CAD build for the part. Positions are in the model's coordinates, mm. A direction names the side the tool comes from. Round coordinates to 2 decimals unless told otherwise and drop trailing zeros. Write each loop counter-clockwise with the first axis right and the second up, starting at its lowest first coordinate (ties: lowest second). Pieces come first, ordered by that corner, then holes. Notation, with made-up numbers: (40, -21.5) - (54, -21.5) arc R31 ccw to (54, 9.5) - close; hole circle Ø8 at (-35.5, -36.75). An arc over 180 degrees is marked (long way). Answer in a Markdown table with one row per item.
```python
from build123d import *

# Parameters (mm, degrees)
PAD_DEPTH         = 20
POCKET_DEPTH      = 6.001
POCKET_DEPTH_BACK = -28.001


with BuildPart() as part:
    # AdditivePipe: sweep along a path in Sketch
    with BuildLine(Plane.XY) as additivepipe_path:
        Line((0, 0), (0, 47))
    # Sketch001 → AdditivePipe (sweep)
    with BuildSketch(Plane.XZ):
        Polygon((-20, 6), (-20, -6), (-16, -6), (-9, -6), (9, -6), (16, -6), (20, -6), (20, 6), (16, 6), (16, 3), (9, 3), (9, 6), (-9, 6), (-9, 3), (-16, 3), (-16, 6), align=None)
    sweep(path=additivepipe_path.line)

    # Sketch002 → Pad (new body, symmetric)
    with BuildSketch(Plane.YZ):
        Polygon((47, 3), (47, 14), (34, 28), (22, 28), (22, 14), (29, 14), (29, 3), align=None)
    extrude(amount=PAD_DEPTH, both=True)

    # Sketch003 → Pocket (cut, two sides)
    with BuildSketch(Plane.XY) as pocket_sk:
        with BuildLine():
            Line((-4.5, 0), (4.5, 0))
            Line((4.5, 0), (4.5, 7))
            ThreePointArc((4.5, 7), (0, 19.361903), (-4.5, 7))
            Line((-4.5, 0), (-4.5, 7))
        make_face()
    extrude(amount=-POCKET_DEPTH, mode=Mode.SUBTRACT)
    extrude(pocket_sk.sketch, amount=-POCKET_DEPTH_BACK, mode=Mode.SUBTRACT)


solid = part.part
```
Q1. Pull direction Z, two halves, no side cores. Call faces 5 (the flat face through (0, 24, -6)), 6 (the flat face through (0, 47, 4)), 7 (the flat face through (13, 15, 3)), 8 (the flat face through (0, 28, 28)): released by +Z, released by -Z, zero draft, split by the parting line, or undercut.
Computed:
| item | result |
|---|---|
| face 5 | released by -Z |
| face 6 | zero draft |
| face 7 | undercut |
| face 8 | released by +Z |
Q2. Saw through at B-B on x = 0. List the corners of the cut face in (y, z).
Computed:
| item | result |
|---|---|
| outline | (19.36, -6) - (47, -6) - (47, 14) - (34, 28) - (22, 28) - (22, 14) - (29, 14) - (29, 6) - (19.36, 6) - close |
Q3. 3-axis set-ups, long thin cutter, end or side, ignore diameter. For faces 1 (the flat face through (4.5, 3, 0)), 2 (the flat face through (18, 15, 6)), 3 (the flat face through (0, 22, 21)), 4 (the flat face through (-9, 15, 5)): which of +Z, -Z, +X, -X, +Y, -Y reach the whole face in a straight line?
Computed:
| item | result |
|---|---|
| face 1 | +Z, -Z, -Y |
| face 2 | +X, -X, -Y |
| face 3 | +Z, +X, -X, -Y |
| face 4 | -Y |
Q4. Flat gauge pins, fed straight in: pin 1 (15.5 mm diameter, centred on x = -7.5, z = 20.5, fed in from -Y); pin 2 (2 mm diameter, centred on x = 11, y = 12.5, fed in from +Z); pin 3 (1 mm diameter, centred on x = -7, y = 13.5, fed in from +Z). Where does each tip first touch, or does it go through?
Computed:
| item | result |
|---|---|
| pin 1 | stops at y = 22 |
| pin 2 | stops at z = 3 |
| pin 3 | stops at z = 6 |
Q5. Saw through at D-D on z = 2. List the corners of the cut face in (x, y).
Computed:
| item | result |
|---|---|
| outline | (-20, 0) - (-4.5, 0) - (-4.5, 7) arc R7 cw (long way) to (4.5, 7) - (4.5, 0) - (20, 0) - (20, 47) - (-20, 47) - close |
Q6. Saw through at C-C on y = 5.5. List the corners of the cut face in (x, z).
Computed:
| item | result |
|---|---|
| outline | (-20, -6) - (-4.5, -6) - (-4.5, 6) - (-9, 6) - (-9, 3) - (-16, 3) - (-16, 6) - (-20, 6) - close; (4.5, -6) - (20, -6) - (20, 6) - (16, 6) - (16, 3) - (9, 3) - (9, 6) - (4.5, 6) - close |
Q7. Saw through at A-A on y = 24. List the corners of the cut face in (x, z).
Computed:
| item | result |
|---|---|
| outline | (-20, -6) - (20, -6) - (20, 6) - (16, 6) - (16, 3) - (9, 3) - (9, 6) - (-9, 6) - (-9, 3) - (-16, 3) - (-16, 6) - (-20, 6) - close; (-20, 14) - (20, 14) - (20, 28) - (-20, 28) - close |
Q8. Drill centre lines: line 1 (Z direction, x = -0.5, y = 26.5); line 2 (X direction, y = 6.5, z = -3); line 3 (X direction, y = 17, z = 3.5). Where is each one in solid material? Low to high.
Computed:
| item | result |
|---|---|
| line 1 | z = -6 to 6, 14 to 28 |
| line 2 | x = -20 to -4.5, 4.5 to 20 |
| line 3 | x = -20 to -16, -9 to -5.24, 5.24 to 9, 16 to 20 |
